Design review of the part built by this model. Coordinates are the model's own, in mm. A direction names the side the tool comes from. Give positions to 0.01 mm unless a question says otherwise; leave off trailing zeros. Write each loop counter-clockwise with the first axis right and the second up, starting at its lowest first coordinate (ties: lowest second). Pieces come first, ordered by that corner, then holes. Notation, with made-up numbers: M 13,76.25 L 60,76.25 A18 ccw 60,86.25 Z; hole C 25,29.5 d9. An arc over 180 degrees is marked long. Answer in a Markdown table with one row per item.
```python
from build123d import *

# Parameters (mm, degrees)
SKETCH1_W           = 6
SKETCH1_H           = 12.5
SKETCH1_W_2         = 15.5
SKETCH1_H_2         = 6
BOSS_EXTRUDE1_DEPTH = 8
CHAMFER1_SIZE       = 1
SKETCH2_R           = 2
CUT_EXTRUDE1_DEPTH  = 6
SKETCH3_R           = 2
CUT_EXTRUDE2_DEPTH  = 7


with BuildPart() as part:
    # Sketch1 → Boss-Extrude1 (new body)
    with BuildSketch(Plane(origin=(0, 0, 0), x_dir=(0, 0, -1), z_dir=(1, 0, 0))):
        with Locations((12.5, 12.25)):
            Rectangle(SKETCH1_W, SKETCH1_H)
        with Locations((7.75, 3)):
            Rectangle(SKETCH1_W_2, SKETCH1_H_2)
    extrude(amount=BOSS_EXTRUDE1_DEPTH)

    # Chamfer1
    chamfer1_edges = [part.edges().sort_by_distance(p)[0] for p in [
        (4, 6, -9.5),
    ]]
    chamfer(chamfer1_edges, length=CHAMFER1_SIZE)

    # Sketch2 → Cut-Extrude1 (cut)
    with BuildSketch(Plane(origin=(0, 0, -15.5), x_dir=(-1, 0, 0), z_dir=(0, 0, -1))):
        with Locations((-4, 14.5)):
            Circle(SKETCH2_R)
        with Locations((-4, 4.5)):
            Circle(SKETCH2_R)
    extrude(amount=-CUT_EXTRUDE1_DEPTH, mode=Mode.SUBTRACT)

    # Sketch3 → Cut-Extrude2 (cut, through all)
    with BuildSketch(Plane(origin=(0, 6, 0), x_dir=(1, 0, 0), z_dir=(0, 1, 0))):
        with Locations((4, 4.5)):
            Circle(SKETCH3_R)
    extrude(amount=-CUT_EXTRUDE2_DEPTH, mode=Mode.SUBTRACT)


solid = part.part
```
1) To check wall thickness, follow probe 1 along Y at (x, z) = (4, -12.5); probe 2 along Z at (x, y) = (4, 1.8); probe 3 along Y at (x, z) = (5.5, -11.25). State the ranges of each line that lie inside material, in increasing order. Write a range as [from, to].
Geometry says:
| item | result |
|---|---|
| probe 1 | [0, 2.5], [6.5, 12.5], [16.5, 18.5] |
| probe 2 | [-15.5, -6.5], [-2.5, 0] |
| probe 3 | [0, 3.18], [5.82, 13.18], [15.82, 18.5] |
2) Add section A-A (x = 4). Write out the cut boundary in (y, z).
Geometry says:
| item | result |
|---|---|
| outline | M 0,-15.5 L 2.5,-15.5 L 2.5,-9.5 L 6.5,-9.5 L 6.5,-15.5 L 12.5,-15.5 L 12.5,-9.5 L 7,-9.5 L 6,-8.5 L 6,-6.5 L 0,-6.5 Z; M 0,-2.5 L 6,-2.5 L 6,0 L 0,0 Z; M 16.5,-15.5 L 18.5,-15.5 L 18.5,-9.5 L 16.5,-9.5 Z |
3) For faces 4 (the face through (5.998, 4.588, -12.542)), 5 (the face through (4.26, 16.483, -12.542)), 6 (the face through (4, 6, -2)), list the 3-axis set-ups (+Z, -Z, +X, -X, +Y, -Y) from which the entire face can be reached by the end or side of a thin tool; tool diameter is ignored.
Geometry says:
| item | result |
|---|---|
| face 4 | -Z |
| face 5 | +Z, -Z |
| face 6 | +Z, +X, -X, +Y |
4) Add section B-B (y = 14.5). Write out the cut boundary in (x, z), and give its area (3 significant figures).
Geometry says:
| item | result |
|---|---|
| outline | M 0,-15.5 L 2,-15.5 L 2,-9.5 L 0,-9.5 Z; M 6,-15.5 L 8,-15.5 L 8,-9.5 L 6,-9.5 Z |
| area | 24.0 mm^2 |
5) Add section C-C (z = -4.5). Write out the cut boundary in (x, y), and give its area (3 significant figures).
Geometry says:
| item | result |
|---|---|
| outline | M 0,0 L 2,0 L 2,6 L 0,6 Z; M 6,0 L 8,0 L 8,6 L 6,6 Z |
| area | 24.0 mm^2 |
6) The part is to be moulded in two halves that separate along X. For faces 1 (the face through (0, 7, -11)), 2 (the face through (3.9, 6.5, -9)), 3 (the face through (2.002, 3.042, -4.588)), say which applies: released by +X, released by -X, zero draft, split by the parting line, or undercut.
Geometry says:
| item | result |
|---|---|
| face 1 | released by -X |
| face 2 | zero draft |
| face 3 | undercut |
7) Add section D-D (y = 2). Write out the cut boundary in (x, z), and give its area (3 significant figures).
Geometry says:
| item | result |
|---|---|
| outline | M 0,-15.5 L 8,-15.5 L 8,0 L 0,0 Z; hole C 4,-4.5 d4 |
| area | 111 mm^2 |
8) Insertion check: P1, Ø2.5, axis at x = 5.5, z = -5, coming from the +Y side; P2, Ø3, axis at x = 4, y = 4.5, coming from the -Z side; P3, Ø4, axis at x = 4, y = 13, coming from the +Z side. Each pin has a flat end and moves straight along its axis. Give the tip position at first contact, or say it passes through.
Geometry says:
| item | result |
|---|---|
| P1 | y = 6 |
| P2 | z = -9.5 |
| P3 | z = -9.5 |
